Work out the finished part from the listing and answer in its coordinate system (mm). A direction names the side the tool comes from. Coordinates: 2 decimals unless noted, no trailing zeros. Write each loop counter-clockwise with the first axis right and the second up, starting at its lowest first coordinate (ties: lowest second). Pieces come first, ordered by that corner, then holes. Notation, with made-up numbers: (-9, 72) - (1, 72) arc R27 cw to (1, 95) - close; hole circle Ø7 at (19.25, -37.75). An arc over 180 degrees is marked (long way). Use a Markdown table: item, result. Add a question column.
(1) For a pull along Z with two mould halves and no side action, classify faces 1 (the face through (-36, 176, 40)), 2 (the face through (-63.835, 164.943, 21.201)), 3 (the face through (46.855, 105.254, 19.72)) as released by +Z, released by -Z, zero draft, split by the parting line, or undercut.
(2) The part is cut by section C-C, the plane z = 22. Give the vertices of the cut face in (x, y).
(3) The part is cut by section D-D, the plane z = 13. Give the vertices of the cut face in (x, y), then the cut area to 3 significant figures.
(4) The part is cut by section A-A, the plane y = 135. Give the vertices of the cut face in (x, z), then the cut area to 3 significant figures.
(5) Find the intervals of material crossed by line 1 (X direction, y = 135, z = 25.5); line 2 (Y direction, x = 0, z = 11); line 3 (Y direction, x = -9.5, z = 25), in increasing order. Write a range as from..to.
(6) Given pin 1 Ø1.5 at (x, z) = (-25, 33) entering from +Y; pin 2 Ø12 at (x, z) = (39, 14) entering from +Y; pin 3 Ø5 at (x, z) = (25, 35) entering from -Y, each flat-ended and moving along its own axis, determine where each tip first touches the part or whether it passes through.
(7) A tool of negligible diameter and unlimited length cuts with its end or side. For faces 4 (the face through (-61.168, 162.232, 15.276)), 5 (the face through (-53.9, 174.2, 15.3)), 6 (the face through (-49.51, 157.01, 19.72)), from which of +Z, -Z, +X, -X, +Y, -Y can it reach the whole face along a straight path? Write none if from no direction.
(8) The part is cut by section B-B, the plane x = 0. Give the vertices of the cut face in (y, z), then the cut area to 3 significant figures.
from build123d import *

# Parameters (mm, degrees)
SM_BASE_FLANGE_1_DEPTH = 40
SKETCH_6_R             = 4
CUT_EXTRUDE_1_DEPTH    = 162.312299626


# Read off the part's stored shape, not the designer's step: Базовая кромка1
with BuildPart() as part:
    # Базовая кромка1 outline → Базовая кромка1 (new body)
    with BuildSketch(Plane.XY):
        with BuildLine():
            Line((-44.739249061, 168.913121258), (-63.336309448, 179.650139078))
            Line((-63.336309448, 179.650139078), (-64.336309448, 177.91808827))
            Line((-64.336309448, 177.91808827), (-45.739249061, 167.18107045))
            ThreePointArc((-45.739249061, 167.18107045), (-43.846610356, 166.865137493), (-42.211758442, 167.869704125))
            ThreePointArc((-42.211758442, 167.869704125), (46.332359104, 108.250000003), (-49.571878008, 155.121603086))
            ThreePointArc((-49.571878008, 155.121603086), (-49.519323742, 157.039709692), (-50.739249061, 158.520816412))
            Line((-50.739249061, 158.520816412), (-69.336309448, 169.257834232))
            Line((-69.336309448, 169.257834232), (-70.336309448, 167.525783425))
            Line((-70.336309448, 167.525783425), (-51.739249061, 156.788765605))
            ThreePointArc((-51.739249061, 156.788765605), (-51.410886498, 156.390101858), (-51.425032326, 155.873812548))
            ThreePointArc((-51.425032326, 155.873812548), (48.064409909, 107.249999999), (-43.789768103, 169.098478111))
            ThreePointArc((-43.789768103, 169.098478111), (-44.229814847, 168.82808281), (-44.739249061, 168.913121258))
        make_face()
    extrude(amount=SM_BASE_FLANGE_1_DEPTH)

    # Эскиз6 → Вырез-Вытянуть1 (cut, through all)
    with BuildSketch(Plane(origin=(61.956714755, 107.312177826, 0), x_dir=(0.8660254037844433, -0.499999999999992, 0), z_dir=(0.499999999999992, 0.8660254037844433, 0))):
        with Locations(Location((-133.938904682, -20, 0), (0, 0, 180))):
            Circle(SKETCH_6_R)
    extrude(amount=-CUT_EXTRUDE_1_DEPTH, mode=Mode.SUBTRACT)


solid = part.part
Model answer:
| question | item | result |
|---|---|---|
| 1 | face 1 | released by +Z |
| 1 | face 2 | undercut |
| 1 | face 3 | zero draft |
| 2 | outline | (-70.34, 167.53) - (-64.04, 163.89) - (-63.04, 165.62) - (-69.34, 169.26) - close; (-64.34, 177.92) - (-58.04, 174.28) - (-57.04, 176.01) - (-63.34, 179.65) - close; (-58.04, 160.43) - (-51.74, 156.79) arc R0.74 cw to (-51.43, 155.87) arc R55.5 ccw (long way) to (-43.79, 169.1) arc R0.74 cw to (-44.74, 168.91) - (-51.04, 172.55) - (-52.04, 170.82) - (-45.74, 167.18) arc R2.74 ccw to (-42.21, 167.87) arc R53.5 cw (long way) to (-49.57, 155.12) arc R2.74 ccw to (-50.74, 158.52) - (-57.04, 162.16) - close |
| 3 | outline | (-70.34, 167.53) - (-51.74, 156.79) arc R0.74 cw to (-51.43, 155.87) arc R55.5 ccw (long way) to (-43.79, 169.1) arc R0.74 cw to (-44.74, 168.91) - (-63.34, 179.65) - (-64.34, 177.92) - (-45.74, 167.18) arc R2.74 ccw to (-42.21, 167.87) arc R53.5 cw (long way) to (-49.57, 155.12) arc R2.74 ccw to (-50.74, 158.52) - (-69.34, 169.26) - close |
| 3 | area | 751 mm^2 |
| 4 | outline | (-55.5, 0) - (-53.5, 0) - (-53.5, 40) - (-55.5, 40) - close; (53.5, 0) - (55.5, 0) - (55.5, 40) - (53.5, 40) - close |
| 4 | area | 160 mm^2 |
| 5 | line 1 | -55.5..-53.5, 53.5..55.5 |
| 5 | line 2 | 79.5..81.5, 188.5..190.5 |
| 5 | line 3 | 80.32..82.35, 187.65..189.68 |
| 6 | pin 1 | y = 184.92 |
| 6 | pin 2 | y = 179.62 |
| 6 | pin 3 | y = 84.27 |
| 7 | face 4 | +Z, -Z, -X |
| 7 | face 5 | +Z, -Z, +Y |
| 7 | face 6 | +Z, -Z |
| 8 | outline | (79.5, 0) - (81.5, 0) - (81.5, 40) - (79.5, 40) - close; (188.5, 0) - (190.5, 0) - (190.5, 40) - (188.5, 40) - close |
| 8 | area | 160 mm^2 |
